Drawing for the job (mm, zero at the part's lowest x, y, z). A direction names the side the tool comes from. Round coordinates to 2 decimals unless told otherwise and drop trailing zeros. Write each loop counter-clockwise with the first axis right and the second up, starting at its lowest first coordinate (ties: lowest second). Pieces come first, ordered by that corner, then holes. Notation, with made-up numbers: (8, 84.25) - (28, 84.25) arc R16 ccw to (28, 97.25) - close; hole circle Ø8 at (81, 85.25). An arc over 180 degrees is marked (long way). One line per question, with ' | ' between items.
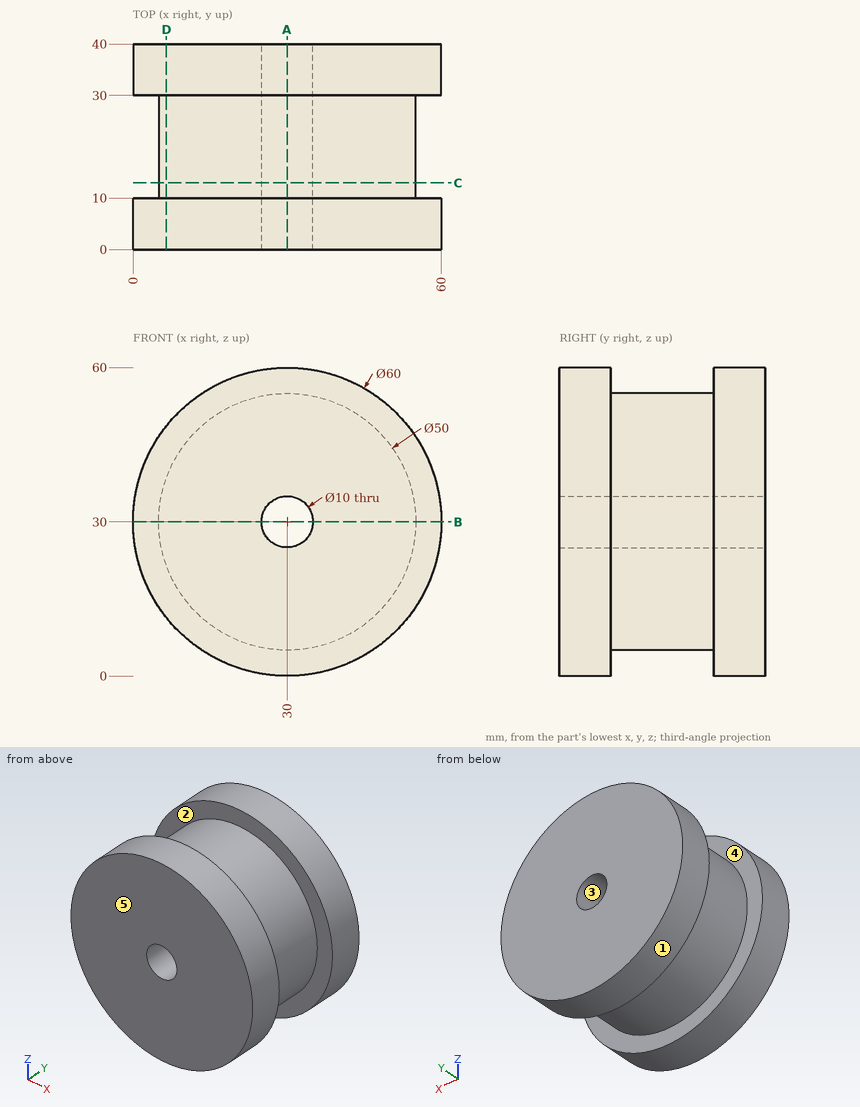
Q1. Saw through at D-D, the plane x = 6.5. List the corners of the cut face in (y, z), then the cut area to 3 significant figures.
Found:
outline: (0, 11.35) - (10, 11.35) - (10, 21.47) - (30, 21.47) - (30, 11.35) - (40, 11.35) - (40, 48.65) - (30, 48.65) - (30, 38.53) - (10, 38.53) - (10, 48.65) - (0, 48.65) - close | area: 1,090 mm^2
Q2. Which spindle directions (+Z, -Z, +X, -X, +Y, -Y) get a long thin tool onto all of the face, cutting with end or side? Do the marked faces 4 and 5. Say none if no direction does.
Found:
face 4: none | face 5: +Z, -Z, +X, -X, -Y
Q3. Saw through at B-B, the plane z = 30. List the corners of the cut face in (x, y).
Found:
outline: (0, 0) - (25, 0) - (25, 40) - (0, 40) - (0, 30) - (5, 30) - (5, 10) - (0, 10) - close; (35, 0) - (60, 0) - (60, 10) - (55, 10) - (55, 30) - (60, 30) - (60, 40) - (35, 40) - close
Q4. Drop flat-ended pins along their axis: pin 1 (8 mm diameter, centred on x = 44, y = 8, fed in from +Z); pin 2 (6 mm diameter, centred on x = 17, y = 10, fed in from -Z); pin 3 (2 mm diameter, centred on y = 33.5, z = 22, fed in from +X). Give the stop position or say it passes through.
Found:
pin 1: z = 58.28 | pin 2: z = 1.72 | pin 3: x = 59.17
Q5. Saw through at A-A, the plane x = 30. List the corners of the cut face in (y, z), then the cut area to 3 significant figures.
Found:
outline: (0, 0) - (10, 0) - (10, 5) - (30, 5) - (30, 0) - (40, 0) - (40, 25) - (0, 25) - close; (0, 35) - (40, 35) - (40, 60) - (30, 60) - (30, 55) - (10, 55) - (10, 60) - (0, 60) - close | area: 1,800 mm^2
Q6. Pull direction X, two halves, no side cores. Call the marked faces 1, 2 and 3: +X half, -X half, draft (parallel to the pull), parting line (faces both ways), or undercut.
Found:
face 1: parting line | face 2: draft | face 3: undercut
Q7. Saw through at C-C, the plane y = 13. List the corners of the cut face in (x, z).
Found:
outline: circle Ø50 at (30, 30); hole circle Ø10 at (30, 30)
Q8. Drill centre lines: L1, parallel to Z at x = 30, y = 22; L2, parallel to Y at x = 46.5, z = 49. Where is each one in solid material? Low to high. Write a range as from..to.
Found:
L1: 5..25, 35..55 | L2: 0..10, 30..40
